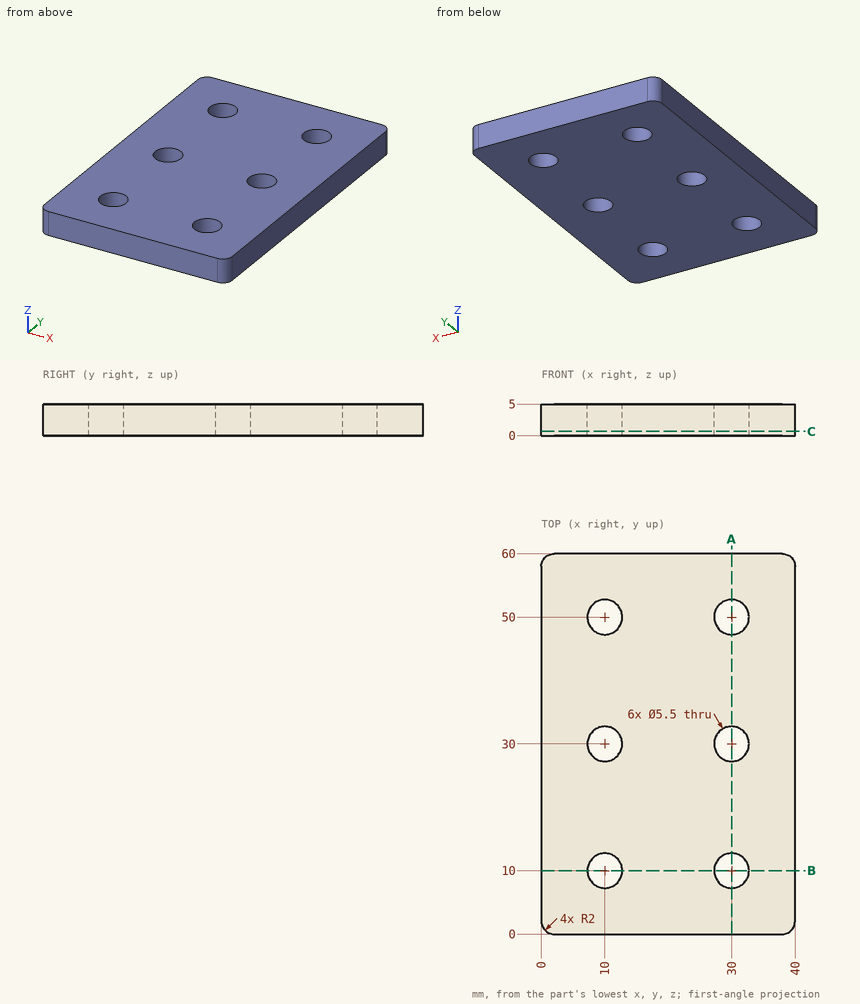
Input: dimensioned drawing with shaded views. Units: mm. Origin: part minimum x, y, z. Round coordinates to 2 decimals unless told otherwise and drop trailing zeros. Order: outer loops, then holes, each group sorted by start corner. A loop starts at its lowest first (then second) coordinate and runs counter-clockwise, first axis right, second up. Notation, with made-up numbers: (-8, 84.25) - (15, 84.25) arc R18 ccw to (15, 118.25) - close; hole circle Ø7 at (80.5, -37). An arc over 180 degrees is marked (long way). Use CSV: the item, a comma, the result in double quotes. Start each with the question number.
Q1. Section query C-C (z = 0.7). Return loops of the section in (x, y).
Q2. Section query B-B (y = 10). Return loops of the section in (x, z), and give its area (3 significant figures).
Q3. Material intervals for line 1 along X through (y, z) = (50, 1.5); line 2 along Y through (x, z) = (10, 1.8); line 3 along X through (y, z) = (48, 1.25), sorted ascending. Write a range as from..to.
Q4. Section query A-A (x = 30). Return loops of the section in (y, z).
Q5. First-contact query: pin 1 (5 mm diameter, centred on x = 30, y = 50, fed in from -Z). Flat tip, straight axial feed; report the tip coordinate or a pass-through.
Result set:
1,outline,"(0, 2) arc R2 ccw to (2, 0) - (38, 0) arc R2 ccw to (40, 2) - (40, 58) arc R2 ccw to (38, 60) - (2, 60) arc R2 ccw to (0, 58) - close; hole circle Ø5.5 at (10, 10); hole circle Ø5.5 at (10, 30); hole circle Ø5.5 at (10, 50); hole circle Ø5.5 at (30, 10); hole circle Ø5.5 at (30, 30); hole circle Ø5.5 at (30, 50)"
2,outline,"(0, 0) - (7.25, 0) - (7.25, 5) - (0, 5) - close; (12.75, 0) - (27.25, 0) - (27.25, 5) - (12.75, 5) - close; (32.75, 0) - (40, 0) - (40, 5) - (32.75, 5) - close"
2,area,"145 mm2"
3,line 1,"x = 0..7.25, 12.75..27.25, 32.75..40"
3,line 2,"y = 0..7.25, 12.75..27.25, 32.75..47.25, 52.75..60"
3,line 3,"x = 0..8.11, 11.89..28.11, 31.89..40"
4,outline,"(0, 0) - (7.25, 0) - (7.25, 5) - (0, 5) - close; (12.75, 0) - (27.25, 0) - (27.25, 5) - (12.75, 5) - close; (32.75, 0) - (47.25, 0) - (47.25, 5) - (32.75, 5) - close; (52.75, 0) - (60, 0) - (60, 5) - (52.75, 5) - close"
5,pin 1,"passes through"
